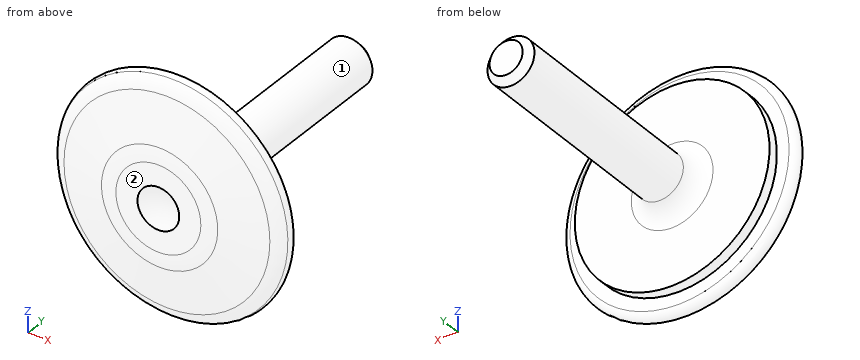
```python
from build123d import *


with BuildPart() as part:
    # Sketch1 → Revolve1 (revolve)
    with BuildSketch(Plane.XY, mode=Mode.PRIVATE) as revolve1_sk:
        with BuildLine():
            Line((3, 0), (6.110643917, 0))
            ThreePointArc((6.110643917, 0), (7.242676055, 0.064281443), (8.36015446, 0.256299352))
            Line((8.36015446, 0.256299352), (14.800032714, 1.743062396))
            ThreePointArc((14.800032714, 1.743062396), (15.788233421, 2.169324212), (16.562410224, 2.916913705))
            ThreePointArc((16.562410224, 2.916913705), (16.639687107, 3.956570753), (15.75, 4.5))
            Line((15.75, 4.5), (14, 4.5))
            Line((14, 4.5), (14, 6))
            Line((14, 6), (5.875, 6))
            ThreePointArc((5.875, 6), (4.107233047, 6.732233047), (3.375, 8.5))
            Line((3.375, 8.5), (3.375, 38.8))
            Line((3.375, 38.8), (2.375, 39.8))
            Line((2.375, 39.8), (0, 39.8))
            Line((0, 39.8), (0, 1))
            ThreePointArc((0, 1), (1.58113883, 0.74341649), (3, 0))
        make_face()
    revolve(revolve1_sk.sketch.rotate(Axis((0, 0, 0), (0, 1, 0)), 90), axis=Axis((0, 0, 0), (0, 1, 0)))


solid = part.part
```
Part model, mm, in its own coordinate system. Face numbers are marked on the shaded views. A direction names the side the tool comes from. Round coordinates to 2 decimals unless told otherwise and drop trailing zeros. Write each loop counter-clockwise with the first axis right and the second up, starting at its lowest first coordinate (ties: lowest second). Pieces come first, ordered by that corner, then holes. Notation, with made-up numbers: (27.5, 18.5) -> (41.5, 18.5) arc R14 cw to (41.5, 41.5) -> close; hole circle Ø5 at (79, -16). An arc over 180 degrees is marked (long way). Return JSON: item names as keys, results as strings. Group by question number.
Q1. Which spindle directions (+Z, -Z, +X, -X, +Y, -Y) get a long thin tool onto all of the face, cutting with end or side? Do the marked faces 1 and 2. Say none if no direction does.
Q2. Pin check, flat tips, straight feed: pin 1 (1.5 mm diameter, centred on y = 4, z = 10, fed in from +X); pin 2 (3 mm diameter, centred on x = 0.5, y = 26, fed in from -Z) (3 decimals); pin 3 (1 mm diameter, centred on x = -8.5, z = -0.5, fed in from +Y); pin 4 (4 mm diameter, centred on x = -5.5, y = 10, fed in from -Z). Stop position of each tip, or through.
Q3. Saw through at A-A on y = 37. Write the cut outline in (x, z) (3 decimals).
Q4. Probe L1, parallel to X at y = 17, z = 0 (3 decimals); L2, parallel to Y at x = -15, z = -4.5; L3, parallel to Y at x = -7, z = -11. List the from-to ranges inside material, lowest first. Write a range as [from, to].
Answer:
{
 "1": {"face 1": "+Y", "face 2": "+Z, -Z, +X, -X, -Y"},
 "2": {"pin 1": "x = 13.9", "pin 2": "z = -3.375", "pin 3": "y = 6", "pin 4": "through"},
 "3": {"outline": "circle Ø6.75 at (0, 0)"},
 "4": {"L1": "[-3.375, 3.375]", "L2": "[2.09, 4.5]", "L3": "[1.34, 6]"}
}
